```python
from build123d import *

# Parameters (mm, degrees)
ESBO_O1_W                = 115
ESBO_O1_H                = 100
RESSALTO_EXTRUS_O1_DEPTH = 1.5
RESSALTO_EXTRUS_O2_DEPTH = 3
ESBO_O2_R                = 1.5
CORTE_EXTRUS_O1_DEPTH    = 4
SKETCH2_W                = 11.7
SKETCH2_H                = 3
CUT_EXTRUDE3_DEPTH       = 2.5
CUT_EXTRUDE3_DEPTH_BACK  = 2.5


with BuildPart() as part:
    # Esboço1 → Ressalto-extrusão1 (new body, symmetric)
    with BuildSketch(Plane(origin=(0, 0, 0), x_dir=(1, 0, 0), z_dir=(0, 1, 0))):
        Rectangle(ESBO_O1_W, ESBO_O1_H)
    extrude(amount=RESSALTO_EXTRUS_O1_DEPTH, both=True)

    # Esboço4 → Ressalto-extrusão2 (add, through all)
    with BuildSketch(Plane(origin=(0, 1.5, 0), x_dir=(1, 0, 0), z_dir=(0, 1, 0))):
        with BuildLine():
            Line((6.5, 53), (20, 53))
            Line((20, 53), (20, 50))
            Line((20, 50), (-20, 50))
            Line((-20, 50), (-20, 53))
            Line((-20, 53), (-6.5, 53))
            ThreePointArc((-6.5, 53), (-5.085786438, 53.585786438), (-4.5, 55))
            Line((-4.5, 55), (-4.5, 55.2))
            ThreePointArc((-4.5, 55.2), (-4.265685425, 55.765685425), (-3.7, 56))
            Line((-3.7, 56), (3.7, 56))
            ThreePointArc((3.7, 56), (4.265685425, 55.765685425), (4.5, 55.2))
            Line((4.5, 55.2), (4.5, 55))
            ThreePointArc((4.5, 55), (5.085786438, 53.585786438), (6.5, 53))
        make_face()
        with BuildLine():
            Line((-63.5, 3.7), (-63.5, -3.7))
            ThreePointArc((-63.5, -3.7), (-63.265685425, -4.265685425), (-62.7, -4.5))
            Line((-62.7, -4.5), (-62.5, -4.5))
            ThreePointArc((-62.5, -4.5), (-61.085786438, -5.085786438), (-60.5, -6.5))
            Line((-60.5, -6.5), (-60.5, -20))
            Line((-60.5, -20), (-57.5, -20))
            Line((-57.5, -20), (-57.5, 20))
            Line((-57.5, 20), (-60.5, 20))
            Line((-60.5, 20), (-60.5, 6.5))
            ThreePointArc((-60.5, 6.5), (-61.085786438, 5.085786438), (-62.5, 4.5))
            Line((-62.5, 4.5), (-62.7, 4.5))
            ThreePointArc((-62.7, 4.5), (-63.265685425, 4.265685425), (-63.5, 3.7))
        make_face()
        with BuildLine():
            Line((4.5, -55.2), (4.5, -55))
            ThreePointArc((4.5, -55), (5.085786438, -53.585786438), (6.5, -53))
            Line((6.5, -53), (20, -53))
            Line((20, -53), (20, -50))
            Line((20, -50), (-20, -50))
            Line((-20, -50), (-20, -53))
            Line((-20, -53), (-6.5, -53))
            ThreePointArc((-6.5, -53), (-5.085786438, -53.585786438), (-4.5, -55))
            Line((-4.5, -55), (-4.5, -55.2))
            ThreePointArc((-4.5, -55.2), (-4.265685425, -55.765685425), (-3.7, -56))
            Line((-3.7, -56), (3.7, -56))
            ThreePointArc((3.7, -56), (4.265685425, -55.765685425), (4.5, -55.2))
        make_face()
        with BuildLine():
            Line((57.5, 20), (60.5, 20))
            Line((60.5, 20), (60.5, 6.5))
            ThreePointArc((60.5, 6.5), (61.085786438, 5.085786438), (62.5, 4.5))
            Line((62.5, 4.5), (62.7, 4.5))
            ThreePointArc((62.7, 4.5), (63.265685425, 4.265685425), (63.5, 3.7))
            Line((63.5, 3.7), (63.5, -3.7))
            ThreePointArc((63.5, -3.7), (63.265685425, -4.265685425), (62.7, -4.5))
            Line((62.7, -4.5), (62.5, -4.5))
            ThreePointArc((62.5, -4.5), (61.085786438, -5.085786438), (60.5, -6.5))
            Line((60.5, -6.5), (60.5, -20))
            Line((60.5, -20), (57.5, -20))
            Line((57.5, -20), (57.5, 20))
        make_face()
    extrude(amount=-RESSALTO_EXTRUS_O2_DEPTH)

    # Esboço2 → Corte-extrusão1 (cut, through all)
    with BuildSketch(Plane(origin=(0, 1.5, 0), x_dir=(1, 0, 0), z_dir=(0, 1, 0))):
        with Locations((0, -51.5)):
            Circle(ESBO_O2_R)
        with Locations((0, 51.5)):
            Circle(ESBO_O2_R)
        with Locations((59, 0)):
            Circle(ESBO_O2_R)
        with Locations((-59, 0)):
            Circle(ESBO_O2_R)
    extrude(amount=-CORTE_EXTRUS_O1_DEPTH, mode=Mode.SUBTRACT)

    # Sketch2 → Cut-Extrude3 (cut, two sides)
    with BuildSketch(Plane(origin=(0, 0, 0), x_dir=(1, 0, 0), z_dir=(0, 1, 0))) as cut_extrude3_sk:
        with Locations((43.4, 23.8)):
            Rectangle(SKETCH2_W, SKETCH2_H)
    extrude(amount=CUT_EXTRUDE3_DEPTH, mode=Mode.SUBTRACT)
    extrude(cut_extrude3_sk.sketch, amount=-CUT_EXTRUDE3_DEPTH_BACK, mode=Mode.SUBTRACT)


solid = part.part
```
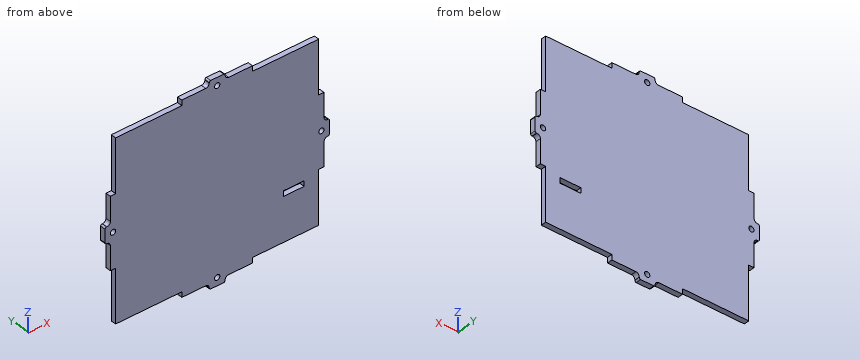
Build history of the part. All positions in model axes, mm. Give positions to 0.01 mm unless a question says otherwise; leave off trailing zeros. Loops run counter-clockwise (first coordinate to the right, second up) from the corner with the lowest first, then second, coordinate; pieces in that order, holes last.
1) Band-saw the part on C-C on y = -0.65. State how many separate pieces and enclosed holes the cut face has, then the cut area to 3 significant figures.
Values follow:
separate pieces: 1
enclosed holes: 5
area: 12,000 mm2
2) Probe line 1 along X through (y, z) = (-0.9, 0); line 2 along Z through (x, y) = (0, -0.75); line 3 along Z through (x, y) = (46, -0.6). List the from-to ranges inside material, lowest first.
Values follow:
line 1: x = -63.5 to -60.5, -57.5 to 57.5, 60.5 to 63.5
line 2: z = -56 to -53, -50 to 50, 53 to 56
line 3: z = -50 to -25.3, -22.3 to 50
3) Band-saw the part on B-B on z = -51.5. List the corners of the cut face in (x, y), then the cut area to 3 significant figures.
Values follow:
outline: (-20, -1.5) - (-1.5, -1.5) - (-1.5, 1.5) - (-20, 1.5) - close; (1.5, -1.5) - (20, -1.5) - (20, 1.5) - (1.5, 1.5) - close
area: 111 mm2
4) Band-saw the part on A-A on x = 40. List the corners of the cut face in (y, z).
Values follow:
outline: (-1.5, -50) - (1.5, -50) - (1.5, -25.3) - (-1.5, -25.3) - close; (-1.5, -22.3) - (1.5, -22.3) - (1.5, 50) - (-1.5, 50) - close
5) Band-saw the part on D-D on z = 29. List the corners of the cut face in (x, y), then the cut area to 3 significant figures.
Values follow:
outline: (-57.5, -1.5) - (57.5, -1.5) - (57.5, 1.5) - (-57.5, 1.5) - close
area: 345 mm2
6) Drop flat-ended pins along their axis: P1, Ø1.5, axis at x = 41, y = -0.5, coming from the -Z side; P2, Ø0.9, axis at y = 0.5, z = 52, coming from the -X side; P3, Ø4, axis at x = 0, z = 51.5, coming from the +Y side; P4, Ø0.9, axis at y = -0.5, z = 39, coming from the +X side. Give the stop position or say it passes through.
Values follow:
P1: stops at z = -50
P2: stops at x = -20
P3: stops at y = 1.5
P4: stops at x = 57.5
